Check sheet for the modelled part. Datum: model origin and axes. Units: mm. A direction names the side the tool comes from. Round coordinates to 2 decimals unless told otherwise and drop trailing zeros. Write each loop counter-clockwise with the first axis right and the second up, starting at its lowest first coordinate (ties: lowest second). Pieces come first, ordered by that corner, then holes. Notation, with made-up numbers: M 47,67.5 L 81,67.5 A31 cw 81,95.5 Z; hole C -1,19 d5. An arc over 180 degrees is marked long. Put each result on its own line as item: value.
```python
from build123d import *

# Parameters (mm, degrees)
SKETCH1_R                = 1
BOSS_EXTRUDE2_DEPTH      = 4
BOSS_EXTRUDE3_DEPTH      = 10
SKETCH3_W                = 26
SKETCH3_H                = 10
CUT_EXTRUDE1_DEPTH       = 10
BOSS_EXTRUDE4_DEPTH      = 26
SKETCH8_W                = 23
SKETCH8_H                = 4
CUT_EXTRUDE5_DEPTH       = 9
SKETCH10_R               = 3
CUT_EXTRUDE7_DEPTH       = 0.7
SKETCH11_R               = 2
CUT_EXTRUDE8_DEPTH       = 10.7
BOSS_EXTRUDE5_START      = -26
BOSS_EXTRUDE5_DEPTH      = 26
SKETCH14_W               = 18
SKETCH14_H               = 1
CUT_EXTRUDE10_DEPTH      = 5
CUT_EXTRUDE11_DEPTH      = 1
CUT_EXTRUDE11_DEPTH_BACK = 5.5
SKETCH15_W               = 18
SKETCH15_H               = 2.914160071
SKETCH16_R               = 1.5
SKETCH16_R_2             = 1
BOSS_EXTRUDE6_DEPTH      = 1
FILLET3_R                = 2
FILLET4_R                = 3


# Read off the part's stored shape, not the designer's step: Boss-Extrude5
with BuildPart() as part:
    # Sketch1 → Boss-Extrude2 (new body)
    with BuildSketch(Plane.XY):
        with BuildLine():
            Line((-18.57209146, 27.379059863), (36.519389128, 27.379059863))
            ThreePointArc((36.519389128, 27.379059863), (50.519389128, 13.379059863), (36.519389128, -0.620940137))
            Line((36.519389128, -0.620940137), (21.833027405, -0.620940137))
            Line((21.833027405, -0.620940137), (21.833027405, -3.648981121))
            Line((21.833027405, -3.648981121), (-4.166972595, -3.648981121))
            Line((-4.166972595, -3.648981121), (-4.166972595, -0.620940137))
            Line((-4.166972595, -0.620940137), (-18.57209146, -0.620940137))
            ThreePointArc((-18.57209146, -0.620940137), (-32.57209146, 13.379059863), (-18.57209146, 27.379059863))
        make_face()
        with Locations((-1.526351166, 20.851018883)):
            Circle(SKETCH1_R, mode=Mode.SUBTRACT)
        with Locations((19.473648834, 20.851018883)):
            Circle(SKETCH1_R, mode=Mode.SUBTRACT)
        with Locations((-1.526351166, 6.851018883)):
            Circle(SKETCH1_R, mode=Mode.SUBTRACT)
        with Locations((19.473648834, 6.851018883)):
            Circle(SKETCH1_R, mode=Mode.SUBTRACT)
    extrude(amount=BOSS_EXTRUDE2_DEPTH)

    # Sketch2 → Boss-Extrude3 (add)
    with BuildSketch(Plane.XY.offset(4)):
        with BuildLine():
            Line((-4.166972595, -0.620940137), (-4.166972595, -0.624002345))
            Line((-4.166972595, -0.624002345), (21.833027405, -0.624002345))
            Line((21.833027405, -0.624002345), (21.833027405, -0.620940137))
            Line((21.833027405, -0.620940137), (36.519389128, -0.620940137))
            ThreePointArc((36.519389128, -0.620940137), (50.519389128, 13.379059863), (36.519389128, 27.379059863))
            Line((36.519389128, 27.379059863), (-18.57209146, 27.379059863))
            ThreePointArc((-18.57209146, 27.379059863), (-32.57209146, 13.379059863), (-18.57209146, -0.620940137))
            Line((-18.57209146, -0.620940137), (-4.166972595, -0.620940137))
        make_face()
        with BuildLine():
            ThreePointArc((-18.57209146, 1.379059863), (-30.57209146, 13.379059863), (-18.57209146, 25.379059863))
            Line((-18.57209146, 25.379059863), (36.519389128, 25.379059863))
            ThreePointArc((36.519389128, 25.379059863), (48.519389128, 13.379059863), (36.519389128, 1.379059863))
            Line((36.519389128, 1.379059863), (-18.57209146, 1.379059863))
        make_face(mode=Mode.SUBTRACT)
    extrude(amount=BOSS_EXTRUDE3_DEPTH)

    # Sketch3 → Cut-Extrude1 (cut)
    with BuildSketch(Plane.XZ.offset(0.624002345)):
        with Locations((8.833027405, 9)):
            Rectangle(SKETCH3_W, SKETCH3_H)
    extrude(amount=-CUT_EXTRUDE1_DEPTH, mode=Mode.SUBTRACT)

    # Sketch4 → Boss-Extrude4 (add)
    with BuildSketch(Plane(origin=(21.833027405, 0, 0), x_dir=(0, 0, -1), z_dir=(1, 0, 0))):
        with BuildLine():
            Line((-4, -3.648981121), (7.0957e-05, -3.648981121))
            add(Edge.make_bspline(
                [(7.0957e-05, -3.648981121), (7.0957e-05, -22.995880537), (14.23768392, -22.995880537)],
                knots=[0, 0, 0, 1, 1, 1], degree=2))
            Line((14.23768392, -22.995880537), (22.23768392, -22.995880537))
            ThreePointArc((22.23768392, -22.995880537), (23.651897483, -23.581666974), (24.23768392, -24.995880537))
            Line((24.23768392, -24.995880537), (24.23768392, -28.620008298))
            ThreePointArc((24.23768392, -28.620008298), (23.651897483, -30.034221861), (22.23768392, -30.620008298))
            Line((22.23768392, -30.620008298), (14.23768392, -30.620008298))
            add(Edge.make_bspline(
                [(-4, -3.648981121), (-3.999929043, -30.620008298), (14.23768392, -30.620008298)],
                knots=[0, 0, 0, 1, 1, 1], degree=2))
        make_face()
    extrude(amount=-BOSS_EXTRUDE4_DEPTH)

    # Sketch8 → Cut-Extrude5 (cut)
    with BuildSketch(Plane(origin=(0, 0, -24.237684184), x_dir=(-1, 0, 0), z_dir=(0, 0, -1))):
        with Locations((-8.833027405, -28.620008644)):
            Rectangle(SKETCH8_W, SKETCH8_H)
    extrude(amount=-CUT_EXTRUDE5_DEPTH, mode=Mode.SUBTRACT)

    # Sketch10 → Cut-Extrude7 (cut)
    with BuildSketch(Plane(origin=(0, -22.995880711, 0), x_dir=(1, 0, 0), z_dir=(0, 1, 0))):
        with Locations(Location((8.833027405, 19.237684184, 0), (0, 0, 270))):
            Circle(SKETCH10_R)
    extrude(amount=-CUT_EXTRUDE7_DEPTH, mode=Mode.SUBTRACT)

    # Sketch11 → Cut-Extrude8 (cut)
    with BuildSketch(Plane(origin=(0, -23.695880711, 0), x_dir=(1, 0, 0), z_dir=(0, 1, 0))):
        with Locations(Location((8.833027405, 19.23768392, 0), (0, 0, 270))):
            Circle(SKETCH11_R)
    extrude(amount=-CUT_EXTRUDE8_DEPTH, mode=Mode.SUBTRACT)

    # Boss-Extrude5 outline → Boss-Extrude5 (add)
    with BuildSketch(Plane(origin=(21.833027405, 0, 0), x_dir=(0, 0, -1), z_dir=(1, 0, 0)).offset(BOSS_EXTRUDE5_START)):
        with BuildLine():
            ThreePointArc((2.392558217, -5.066956781), (1.80677178, -3.652743218), (0.392558217, -3.066956781))
            Line((0.392558217, -3.066956781), (-1, -3.066956781))
            Line((-1, -3.066956781), (-1, -3.648981121))
            Line((-1, -3.648981121), (7.0828e-05, -3.648981121))
            add(Edge.make_bspline(
                [(0.828692106, -11.857711885), (7.0827e-05, -8.316335967), (7.0828e-05, -3.648981121)],
                knots=[0.758754376, 0.758754376, 0.758754376, 1, 1, 1], degree=2))
            Line((0.828692106, -11.857711885), (2.392558217, -11.857711885))
            Line((2.392558217, -11.857711885), (2.392558217, -5.066956781))
        make_face()
    extrude(amount=BOSS_EXTRUDE5_DEPTH)

    # Sketch14 → Cut-Extrude10 (cut)
    with BuildSketch(Plane.XZ.offset(11.857711885)):
        with Locations((8.833027405, -1.328692104)):
            Rectangle(SKETCH14_W, SKETCH14_H)
    extrude(amount=-CUT_EXTRUDE10_DEPTH, mode=Mode.SUBTRACT)

    # Sketch15 → Cut-Extrude11 (cut, two sides: drawn at the far end of the back side and taken through both)
    with BuildSketch(Plane(origin=(0, 0, -0.828692104), x_dir=(-1, 0, 0), z_dir=(0, 0, -1)).offset(-CUT_EXTRUDE11_DEPTH_BACK)):
        with Locations((-8.833027405, -6.524036817)):
            Rectangle(SKETCH15_W, SKETCH15_H)
    extrude(amount=CUT_EXTRUDE11_DEPTH + CUT_EXTRUDE11_DEPTH_BACK, mode=Mode.SUBTRACT)

    # Sketch16 → Boss-Extrude6 (add)
    # profile 1 of 4: a face of its own
    with BuildSketch(Plane.XY.offset(4)):
        with Locations((-1.526351166, 20.851018883)):
            Circle(SKETCH16_R)
        with Locations((-1.526351166, 20.851018883)):
            Circle(SKETCH16_R_2, mode=Mode.SUBTRACT)
    # profile 2 of 4: a face of its own
    with BuildSketch(Plane.XY.offset(4)):
        with Locations((-1.526351166, 6.851018883)):
            Circle(SKETCH16_R)
        with Locations((-1.526351166, 6.851018883)):
            Circle(SKETCH16_R_2, mode=Mode.SUBTRACT)
    # profile 3 of 4: a face of its own
    with BuildSketch(Plane.XY.offset(4)):
        with Locations((19.473648834, 20.851018883)):
            Circle(SKETCH16_R)
        with Locations((19.473648834, 20.851018883)):
            Circle(SKETCH16_R_2, mode=Mode.SUBTRACT)
    # profile 4 of 4: a face of its own
    with BuildSketch(Plane.XY.offset(4)):
        with Locations((19.473648834, 6.851018883)):
            Circle(SKETCH16_R)
        with Locations((19.473648834, 6.851018883)):
            Circle(SKETCH16_R_2, mode=Mode.SUBTRACT)
    extrude(amount=BOSS_EXTRUDE6_DEPTH)

    # Fillet3
    fillet3_edges = [part.edges().sort_by_distance(p)[0] for p in [
        (50.519389128, 13.379059863, 0),
        (29.176208267, -0.620940137, 0),
        (-11.369532027, -0.620940137, 0),
        (-32.57209146, 13.379059863, 0),
        (8.973648834, 27.379059863, 0),
    ]]
    fillet(fillet3_edges, radius=FILLET3_R)

    # Fillet4
    fillet4_edges = [part.edges().sort_by_distance(p)[0] for p in [
        (8.833027405, -7.981116852, -0.828692104),
    ]]
    fillet(fillet4_edges, radius=FILLET4_R)


solid = part.part
```
1. Cross-section at A-A (x = -7). Enter the section's corners in (y, z).
Computed values:
outline: M -0.62,2 A2 ccw 1.38,0 L 25.38,0 A2 ccw 27.38,2 L 27.38,14 L 25.38,14 L 25.38,4 L 1.38,4 L 1.38,14 L -0.62,14 Z
2. Access from +Z, -Z, +X, -X, +Y, -Y to the whole of each face (thin tool, end or side, straight path). Record for faces 1 (the flat face through (17.833, -8, 0)), 2 (the cylindrical face through (29.07, -0.02, 0.57)), 3 (the flat face through (29, -0.621, 8)), 4 (the flat face through (-11, 1.379, 9)), 5 (the flat face through (9, -29, -15.238)).
Computed values:
face 1: none
face 2: -Z, +X, -Y
face 3: +Z, -Z, +X, -Y
face 4: +Z
face 5: -Z, -Y
3. Scan lines: probe 1 along X at (y, z) = (-13, 2.5); probe 2 along Z at (x, y) = (21, 18.5); probe 3 along Y at (x, z) = (-2.5, 10). Record each from-to range of solid material in increasing order.
Computed values:
probe 1: x = -4.17 to 21.83
probe 2: z = 0 to 4
probe 3: y = 25.38 to 27.38
4. Release check for a two-part mould opening along Y. For faces 6 (the cylindrical face through (-32.57, 13.69, 7.92)), 7 (the cylindrical face through (9.36, 26.78, 0.57)), 8 (the flat face through (8, 14, 4)) record: +Y half, -Y half, draft (parallel to the pull), parting line (faces both ways), or undercut.
Computed values:
face 6: parting line
face 7: +Y half
face 8: undercut
5. Cross-section at D-D (y = -1.5). Enter the section's corners in (x, z).
Computed values:
outline: M -4.17,0 L 21.83,0 L 21.83,4 L -4.17,4 Z
6. Cross-section at B-B (z = -20). Enter the section's corners in (x, y), then the cut area to 3 significant figures.
Computed values:
outline: M -4.17,-30.62 L -2.67,-30.62 L -2.67,-26.62 L 6.98,-26.62 L 6.98,-23.7 L 5.93,-23.7 L 5.93,-23 L -4.17,-23 Z; M 10.68,-26.62 L 20.33,-26.62 L 20.33,-30.62 L 21.83,-30.62 L 21.83,-23 L 11.73,-23 L 11.73,-23.7 L 10.68,-23.7 Z
area: 91.4 mm2
7. Depth check by flat-ended pin: pin 1 Ø2.5 at (x, z) = (10.5, -16.5) entering from +Y; pin 2 Ø2 at (x, y) = (24, 14.5) entering from -Z; pin 3 Ø0.5 at (x, z) = (3.5, -2) entering from -Y; pin 4 Ø9.5 at (x, z) = (8.83, -19.24) entering from -Y. Enter the tip coordinate at first touch or a pass-through.
Computed values:
pin 1: stops at y = -23
pin 2: stops at z = 0
pin 3: stops at y = -25.98
pin 4: stops at y = -30.62
8. Cross-section at C-C (z = 6.5). Enter the section's corners in (x, y).
Computed values:
outline: M -18.57,-0.62 L -4.17,-0.62 L -4.17,1.38 L -18.57,1.38 A12 cw -18.57,25.38 L 36.52,25.38 A12 cw 36.52,1.38 L 21.83,1.38 L 21.83,-0.62 L 36.52,-0.62 A14 ccw 36.52,27.38 L -18.57,27.38 A14 ccw Z
